```python
from build123d import *

# Parameters (mm, degrees)
F0_W     = 50.797824
F0_H     = 31.739995
F1_DEPTH = 31.75
F3_DEPTH = 31.751
F5_DEPTH = 19.05
F7_DEPTH = 31.742131
F9_DEPTH = 19.05


with BuildPart() as f1:
    # F0 (on Front) → F1 (new body)
    with BuildSketch(Plane.XZ):
        with Locations((25.398912, 15.869997)):
            Rectangle(F0_W, F0_H)
    extrude(amount=F1_DEPTH)

    # F2 (on face) → F3 (cut, through all)
    with BuildSketch(Plane.XZ.offset(31.75)):
        Polygon((50.797824, 31.739995), (38.095411, 31.739995), (50.797824, 12.707176), align=None)
    extrude(amount=-F3_DEPTH, mode=Mode.SUBTRACT)

    # F4 (on face) → F5 (cut)
    with BuildSketch(Plane.XZ.offset(31.75)):
        Polygon((31.741131, 12.707176), (50.797824, 12.707176), (38.095411, 31.739995), (31.741131, 31.739995), align=None)
    extrude(amount=-F5_DEPTH, mode=Mode.SUBTRACT)

    # F6 (on face) → F7 (cut, through all)
    with BuildSketch(Plane.YZ.offset(31.741131)):
        Polygon((-31.75, 12.707176), (-12.7, 31.739995), (-31.75, 31.739995), align=None)
    extrude(amount=-F7_DEPTH, mode=Mode.SUBTRACT)

    # F8 (on face) → F9 (cut)
    with BuildSketch(Plane(origin=(0, 0, 0), x_dir=(0, -1, 0), z_dir=(-1, 0, 0))):
        Polygon((12.7, 12.707176), (31.75, 12.707176), (12.7, 31.739995), align=None)
    extrude(amount=-F9_DEPTH, mode=Mode.SUBTRACT)


solid = f1.part
```
Verification items for the finished model (mm, model axes). A direction names the side the tool comes from. Coordinates: 2 decimals unless noted, no trailing zeros. Loops run counter-clockwise (first coordinate to the right, second up) from the corner with the lowest first, then second, coordinate; pieces in that order, holes last. Notation, with made-up numbers: (3, 89) -> (41, 89) arc R29 ccw to (41, 118) -> close; hole circle Ø10 at (-9, 44). An arc over 180 degrees is marked (long way). Answer in a Markdown table with one row per item.
1) Section check D-D (y = -26). Record the cut outline in (x, z), and give its area (3 significant figures).
The answers:
| item | result |
|---|---|
| outline | (0, 0) -> (50.8, 0) -> (50.8, 12.71) -> (31.74, 12.71) -> (31.74, 18.45) -> (19.05, 18.45) -> (19.05, 12.71) -> (0, 12.71) -> close |
| area | 718 mm2 |
2) Depth check by flat-ended pin: P1, Ø15, axis at x = 9.5, y = -23.5, coming from the +Z side; P2, Ø1.5, axis at y = -4, z = 21, coming from the +X side; P3, Ø15, axis at x = 39.5, z = 26.5, coming from the -Y side. Enter the tip coordinate at first touch or a pass-through.
The answers:
| item | result |
|---|---|
| P1 | stops at z = 12.71 |
| P2 | stops at x = 45.76 |
| P3 | stops at y = -12.7 |
3) Section check A-A (y = -8.5). Record the cut outline in (x, z).
The answers:
| item | result |
|---|---|
| outline | (0, 0) -> (50.8, 0) -> (50.8, 12.71) -> (38.1, 31.74) -> (0, 31.74) -> close |
4) Section check B-B (x = 20). Record the cut outline in (y, z), and give its area (3 significant figures).
The answers:
| item | result |
|---|---|
| outline | (-31.75, 0) -> (0, 0) -> (0, 31.74) -> (-12.7, 31.74) -> (-31.75, 12.71) -> close |
| area | 826 mm2 |
5) Scan lines: line 1 along Z through (x, y) = (8, -20.5); line 2 along Y through (x, z) = (2, 14.5); line 3 along X through (y, z) = (-20, 13). Record each from-to range of solid material in increasing order. Write a range as from..to.
The answers:
| item | result |
|---|---|
| line 1 | z = 0..12.71 |
| line 2 | y = -12.7..0 |
| line 3 | x = 19.05..31.74 |
6) Access from +Z, -Z, +X, -X, +Y, -Y to the whole of each face (thin tool, end or side, straight path). Record for faces 1 (the face through (19.05, -18, 18)), 2 (the face through (19, -6, 31.74)), 3 (the face through (31.741, -18, 18)).
The answers:
| item | result |
|---|---|
| face 1 | +Z, -X, -Y |
| face 2 | +Z, +X, -X, +Y, -Y |
| face 3 | +Z, +X, -Y |
7) Section check C-C (z = 28.5). Record the cut outline in (x, y).
The answers:
| item | result |
|---|---|
| outline | (0, -12.7) -> (19.05, -12.7) -> (19.05, -15.94) -> (31.74, -15.94) -> (31.74, -12.7) -> (40.26, -12.7) -> (40.26, 0) -> (0, 0) -> close |
